from build123d import *

# Parameters (mm, degrees)
SKETCH1_R           = 1.5
BOSS_EXTRUDE1_DEPTH = 3
FILLET1_R           = 3
FILLET2_R           = 6


with BuildPart() as part:
    # Sketch1 → Boss-Extrude1 (new body)
    with BuildSketch(Plane(origin=(0, 0, 0), x_dir=(1, 0, 0), z_dir=(0, 1, 0))):
        with BuildLine():
            Line((-42.5, -3), (-42.5, -28))
            Line((-42.5, -28), (22.5, -28))
            Line((22.5, -28), (22.5, -3))
            Line((22.5, -3), (-1.251145888, -3))
            ThreePointArc((-1.251145888, -3), (-13.25, -9.65), (-25.248854112, -3))
            Line((-25.248854112, -3), (-42.5, -3))
        make_face()
        with Locations((-39, -24.5)):
            Circle(SKETCH1_R, mode=Mode.SUBTRACT)
        with BuildLine():
            ThreePointArc((-24.202730122, -6.452730122), (-22.405460244, -8.25), (-24.202730122, -10.047269878))
            Line((-24.202730122, -10.047269878), (-27.797269878, -10.047269878))
            ThreePointArc((-27.797269878, -10.047269878), (-29.594539756, -8.25), (-27.797269878, -6.452730122))
            Line((-27.797269878, -6.452730122), (-24.202730122, -6.452730122))
        make_face(mode=Mode.SUBTRACT)
        with Locations((19, -24.5)):
            Circle(SKETCH1_R, mode=Mode.SUBTRACT)
        with BuildLine():
            ThreePointArc((-2.297269878, -10.047269878), (-4.094539756, -8.25), (-2.297269878, -6.452730122))
            Line((-2.297269878, -6.452730122), (1.297269878, -6.452730122))
            ThreePointArc((1.297269878, -6.452730122), (3.094539756, -8.25), (1.297269878, -10.047269878))
            Line((1.297269878, -10.047269878), (-2.297269878, -10.047269878))
        make_face(mode=Mode.SUBTRACT)
    extrude(amount=BOSS_EXTRUDE1_DEPTH)

    # Fillet1
    fillet1_edges = [part.edges().sort_by_distance(p)[0] for p in [
        (22.5, 1.5, 28),
        (-42.5, 1.5, 28),
    ]]
    fillet(fillet1_edges, radius=FILLET1_R)

    # Fillet2
    fillet2_edges = [part.edges().sort_by_distance(p)[0] for p in [
        (-1.251145888, 1.5, 3),
        (22.5, 1.5, 3),
        (-42.5, 1.5, 3),
        (-25.248854112, 1.5, 3),
    ]]
    fillet(fillet2_edges, radius=FILLET2_R)


solid = part.part
Read the model definition and answer for the solid it produces. Units are mm, in the model's axes. A direction names the side the tool comes from. Round coordinates to 2 decimals unless told otherwise and drop trailing zeros. Loops run counter-clockwise (first coordinate to the right, second up) from the corner with the lowest first, then second, coordinate; pieces in that order, holes last.
Q1. Section C-C on x = -10 is taken. Write down the section's boundary in (y, z).
Q2. Section A-A on y = 1 is taken. Write down the section's boundary in (x, z), and give its area (3 significant figures).
Q3. Section B-B on z = 8.25 is taken. Write down the section's boundary in (x, y), and give its area (3 significant figures).
Q4. Each of these flat-tipped pins is pushed along its axis until it touches: pin 1 (1 mm diameter, centred on x = -7, z = 6, fed in from +Y); pin 2 (0.9 mm diameter, centred on x = 0.5, y = 1, fed in from -Z). Where does it stop, or does it pass through?
Q5. Consider probe 1 along X at (y, z) = (1, 24.5); probe 2 along Z at (x, y) = (-3, 1.65) (3 decimals); probe 3 along X at (y, z) = (2.75, 6). Determine where each line is inside the solid, lowest interval first.
Q6. Determine the mould class of faces 4 (the face through (0, 1, 10.047)), 5 (the face through (22.5, 1, 17)), 6 (the face through (-26, 1, 6.453)), 7 (the face through (-32, 1, 3)) for opening direction Z: released by +Z, released by -Z, zero draft, split by the parting line, or undercut.
Q7. Which of the six approach directions +Z, -Z, +X, -X, +Y, -Y give full straight-line access (tool end or side, diameter ignored) to faces 1 (the face through (3.094, 1.479, 8.21)), 2 (the face through (-10, 0, 15)), 3 (the face through (-0.76, 1.52, 3.53))?
Output:
1. outline: (0, 9.27) - (3, 9.27) - (3, 28) - (0, 28) - close
2. outline: (-42.5, 9) arc R6 ccw to (-36.5, 3) - (-28.21, 3) arc R6 ccw to (-23.75, 4.98) arc R14.15 cw to (-2.75, 4.98) arc R6 ccw to (1.71, 3) - (16.5, 3) arc R6 ccw to (22.5, 9) - (22.5, 25) arc R3 ccw to (19.5, 28) - (-39.5, 28) arc R3 ccw to (-42.5, 25) - close; hole circle Ø3 at (-39, 24.5); hole (-27.8, 6.45) - (-24.2, 6.45) arc R1.8 ccw to (-24.2, 10.05) - (-27.8, 10.05) arc R1.8 ccw to start; hole (-2.3, 6.45) - (1.3, 6.45) arc R1.8 ccw to (1.3, 10.05) - (-2.3, 10.05) arc R1.8 ccw to start; hole circle Ø3 at (19, 24.5)
2. area: 1,430 mm2
3. outline: (-42.45, 0) - (-29.59, 0) - (-29.59, 3) - (-42.45, 3) - close; (-22.41, 0) - (-19.39, 0) - (-19.39, 3) - (-22.41, 3) - close; (-7.11, 0) - (-4.09, 0) - (-4.09, 3) - (-7.11, 3) - close; (3.09, 0) - (22.45, 0) - (22.45, 3) - (3.09, 3) - close
3. area: 115 mm2
4. pin 1: passes through
4. pin 2: stops at z = 3.05
5. probe 1: x = -42.5 to -40.5, -37.5 to 17.5, 20.5 to 22.5
5. probe 2: z = 5.255 to 6.596, 9.904 to 28
5. probe 3: x = -41.7 to -22.74, -3.76 to 21.7
6. face 4: undercut
6. face 5: zero draft
6. face 6: undercut
6. face 7: released by -Z
7. face 1: +Y, -Y
7. face 2: +Z, -Z, +X, -X, -Y
7. face 3: -Z, +Y, -Y
